```python
from build123d import *

# Parameters (mm, degrees)
BOSS_EXTRU_1_DEPTH = 10


with BuildPart() as part:
    # Esquisse1 → Boss.-Extru.1 (new body)
    with BuildSketch(Plane(origin=(0, 0, 0), x_dir=(0, 0, -1), z_dir=(1, 0, 0))):
        Polygon((0, 0), (35.194411003, 0), (32.606220552, 9.659258263), (18.117333157, 5.776972586), (0, 73.391780427), align=None)
    extrude(amount=BOSS_EXTRU_1_DEPTH)


solid = part.part
```
Check sheet for the modelled part. Datum: model origin and axes. Units: mm. A direction names the side the tool comes from. Coordinates: 2 decimals unless noted, no trailing zeros. Order: outer loops, then holes, each group sorted by start corner. A loop starts at its lowest first (then second) coordinate and runs counter-clockwise, first axis right, second up. Notation, with made-up numbers: M -25.75,75.25 L -0.75,75.25 A23 cw -0.75,89.25 Z; hole C -38.75,75.25 d8. An arc over 180 degrees is marked long. One line per question, with ' | ' between items. Start each with the question number.
Item 1: Material ranges on line 1 (Z direction, x = 3, y = 33); line 2 (Z direction, x = 8.5, y = 11); line 3 (Y direction, x = 5.75, z = -22), recorded low to high.
Item 2: Sectioned sample at C-C on y = 37.5. Record the cut outline in (x, z), and give its area (3 significant figures).
Item 3: Gauge pin test, flat end, axial feed: P1, Ø6, axis at x = 7.5, z = -4.5, coming from the -Y side. Record the tip position at first contact, or that the pin passes through.
Item 4: Access from +Z, -Z, +X, -X, +Y, -Y to the whole of each face (thin tool, end or side, straight path). Record for faces 1 (the flat face through (4.93, 7.745, -25.463)), 2 (the flat face through (5, 37, 0)).
Item 5: Sectioned sample at A-A on x = 3.5. Record the cut outline in (y, z).
Item 6: Sectioned sample at B-B on z = -15. Record the cut outline in (x, y).
Answer below:
1) line 1: z = -10.82 to 0 | line 2: z = -16.72 to 0 | line 3: y = 0 to 6.82
2) outline: M 0,-9.62 L 10,-9.62 L 10,0 L 0,0 Z | area: 96.2 mm^2
3) P1: stops at y = 0
4) face 1: +X, -X, +Y | face 2: +Z, +X, -X, +Y, -Y
5) outline: M 0,-35.19 L 9.66,-32.61 L 5.78,-18.12 L 73.39,0 L 0,0 Z
6) outline: M 0,0 L 10,0 L 10,17.41 L 0,17.41 Z
